```python
from build123d import *

# Parameters (mm, degrees)
F1_DEPTH = 4
F2_R     = 15
F3_ANGLE = 2
F5_DEPTH = 4
F7_R     = 90


with BuildPart() as f1:
    # F0 (on Top) → F1 (new body)
    with BuildSketch(Plane.XY):
        Polygon((0, -64.8374632001), (0, -54.8374632001), (-2, -49.8374632001), (-2, 27.1625367999), (-6, 27.1625367999), (-4.0681642161, -57.8382376935), align=None)
    extrude(amount=F1_DEPTH)

    # F2
    f2_edges = [f1.edges().sort_by_distance(p)[0] for p in [
        (-4.068164, -57.838238, 2),
        (-2, -49.837463, 2),
    ]]
    fillet(f2_edges, radius=F2_R)


with BuildPart() as f1_1:
    # F3: moved
    add(f1.part.rotate(Axis((-2, 27.1625367999, 2), (0, 0, -1)), F3_ANGLE))

    # F4 (on face) → F5 (join)
    with BuildSketch(Plane(origin=(0, 0, 0), x_dir=(1, 0, 0), z_dir=(0, 0, -1))):
        with BuildLine():
            Line((-2, -47.1625367999), (-2, -27.1625367999))
            Line((-2, -27.1625367999), (-5.9975633081, -27.3021347867))
            Line((-5.9975633081, -27.3021347867), (-5.9975633081, -47.1625367999))
            Line((-5.9975633081, -47.1625367999), (-1, -72.1625367999))
            ThreePointArc((-1, -72.1625367999), (-0.7071067812, -72.8696435811), (0, -73.1625367999))
            Line((0, -73.1625367999), (0, -49.1625367999))
            ThreePointArc((0, -49.1625367999), (-1.4142135624, -48.5767503623), (-2, -47.1625367999))
        make_face()
    extrude(amount=-F5_DEPTH)

    # F6: F1 across plane


with BuildPart() as f1_2:
    add(f1_1.part)
    add(f1_1.part.mirror(Plane.YZ))

    # F7
    f7_edges = [f1_2.edges().sort_by_distance(p)[0] for p in [
        (-5.997563, 47.162537, 2),
        (5.997563, 47.162537, 2),
    ]]
    fillet(f7_edges, radius=F7_R)


solid = f1_2.part
```
Check sheet for the modelled part. Datum: model origin and axes. Units: mm. A direction names the side the tool comes from. Give positions to 0.01 mm unless a question says otherwise; leave off trailing zeros. Order: outer loops, then holes, each group sorted by start corner. A loop starts at its lowest first (then second) coordinate and runs counter-clockwise, first axis right, second up. Notation, with made-up numbers: M 5,32 L 19,32 A19 cw 19,43 Z; hole C 9,85.5 d6. An arc over 180 degrees is marked long. Answer in a Markdown table with one row per item. Add a question column.
Q1. Thickness scan on L1, parallel to X at y = -33, z = 0.7; L2, parallel to X at y = 0.5, z = 2.9; L3, parallel to X at y = 63, z = 1.25. Record the ranges inside material, lowest first.
Q2. Sectioned sample at B-B, the plane z = 0.65. Record the boundary of the cut face in (x, y), and give its area (3 significant figures).
Q3. Release check for a two-part mould opening along Y. For faces 1 (the flat face through (3.28, -53.7, 1.97)), 2 (the flat face through (-3.28, -53.7, 1.97)), 3 (the flat face through (-4.226, -62.958, 1.972)), 4 (the flat face through (-5.998, 33, 2)) record: released by +Y, released by -Y, zero draft, split by the parting line, or undercut.
Q4. Sectioned sample at A-A, the plane y = 10. Record the boundary of the cut face in (x, z).
Q5. Gauge pin test, flat ends, axial feed: pin 1 Ø1.5 at (y, z) = (-44, 1.5) entering from -X; pin 2 Ø1 at (y, z) = (-26.5, 1) entering from +X; pin 3 Ø2 at (y, z) = (-15, 2.5) entering from -X. Record the tip position at first contact, or that the pin passes through.
Q6. Access from +Z, -Z, +X, -X, +Y, -Y to the whole of each face (thin tool, end or side, straight path). Record for faces 5 (the flat face through (5.998, 33, 2)), 6 (the flat face through (2, 37, 2)), 7 (the cylindrical face through (-5.57, 47, 2.03)).
Q7. Sectioned sample at C-C, the plane y = -37. Record the boundary of the cut face in (x, z), and give its area (3 significant figures).
Verdict:
| question | item | result |
|---|---|---|
| 1 | L1 | -6.73 to -4.1, 4.1 to 6.73 |
| 1 | L2 | -6.32 to -2.93, 2.93 to 6.32 |
| 1 | L3 | -2.83 to 2.83 |
| 2 | outline | M -6.99,-53.85 A15 ccw -5.21,-61.12 L -3.21,-64.85 L -2.86,-54.86 L -3.71,-52.51 A15 cw -4.59,-46.9 L -2,27.16 L -2,47.16 A2 cw 2,47.16 L 2,27.16 L 4.59,-46.9 A15 cw 3.71,-52.51 L 2.86,-54.86 L 3.21,-64.85 L 5.21,-61.12 A15 ccw 6.99,-53.85 L 6,27.3 L 6,38.26 A90 ccw 4.25,55.9 L 1,72.16 A1 ccw -1,72.16 L -4.25,55.9 A90 ccw -6,38.26 L -6,27.3 Z |
| 2 | area | 889 mm² |
| 3 | face 1 | undercut |
| 3 | face 2 | undercut |
| 3 | face 3 | released by -Y |
| 3 | face 4 | zero draft |
| 4 | outline | M -6.21,0 L -2.6,0 L -2.6,4 L -6.21,4 Z; M 2.6,0 L 6.21,0 L 6.21,4 L 2.6,4 Z |
| 5 | pin 1 | x = -6.88 |
| 5 | pin 2 | x = 6.66 |
| 5 | pin 3 | x = -6.53 |
| 6 | face 5 | +Z, -Z, +X, +Y |
| 6 | face 6 | +Z, -Z, -Y |
| 6 | face 7 | +Z, -Z, -X, +Y |
| 7 | outline | M -6.78,0 L -4.24,0 L -4.24,4 L -6.78,4 Z; M 4.24,0 L 6.78,0 L 6.78,4 L 4.24,4 Z |
| 7 | area | 20.3 mm² |
